Source: CAD feature listing. Evaluate the final solid. Frame: model axes, mm. Face numbers are marked on the shaded views. A direction names the side the tool comes from. Coordinates: 2 decimals unless noted, no trailing zeros. Loops run counter-clockwise (first coordinate to the right, second up) from the corner with the lowest first, then second, coordinate; pieces in that order, holes last.
```python
from build123d import *

# Parameters (mm, degrees)
SM_BASE_FLANGE_1_DEPTH            = 5
SM_EDGE_FLANGE_1_STRIP_W          = 26
SM_EDGE_FLANGE_1_STRIP_H          = 5
SM_EDGE_FLANGE_1_STRIP_CUT_DEPTH  = 45
SM_EDGE_FLANGE_1_RELIEF_W         = 28.5
SM_EDGE_FLANGE_1_RELIEF_H         = 2.5
SM_EDGE_FLANGE_1_RELIEF_CUT_DEPTH = 5
SM_EDGE_FLANGE_1_DEPTH            = 45
SM_EDGE_FLANGE_2_STRIP_W          = 26
SM_EDGE_FLANGE_2_STRIP_H          = 5
SM_EDGE_FLANGE_2_STRIP_CUT_DEPTH  = 45
SM_EDGE_FLANGE_2_RELIEF_W         = 28.5
SM_EDGE_FLANGE_2_RELIEF_H         = 2.5
SM_EDGE_FLANGE_2_RELIEF_CUT_DEPTH = 5
SM_EDGE_FLANGE_2_DEPTH            = 45
SM_EDGE_FLANGE_14_DEPTH           = 40
SM_EDGE_FLANGE_15_DEPTH           = 40
SM_EDGE_FLANGE_16_DEPTH           = 40
SM_EDGE_FLANGE_17_DEPTH           = 40
SM_EDGE_FLANGE_18_STRIP_W         = 26
SM_EDGE_FLANGE_18_STRIP_H         = 5
SM_EDGE_FLANGE_18_STRIP_CUT_DEPTH = 40
SM_EDGE_FLANGE_18_DEPTH           = 40
SM_EDGE_FLANGE_19_STRIP_W         = 26
SM_EDGE_FLANGE_19_STRIP_H         = 5
SM_EDGE_FLANGE_19_STRIP_CUT_DEPTH = 40
SM_EDGE_FLANGE_19_DEPTH           = 40
SM_EDGE_FLANGE_20_STRIP_W         = 26
SM_EDGE_FLANGE_20_STRIP_H         = 5
SM_EDGE_FLANGE_20_STRIP_CUT_DEPTH = 40
SM_EDGE_FLANGE_20_DEPTH           = 40
SM_EDGE_FLANGE_21_STRIP_W         = 26
SM_EDGE_FLANGE_21_STRIP_H         = 5
SM_EDGE_FLANGE_21_STRIP_CUT_DEPTH = 40
SM_EDGE_FLANGE_21_DEPTH           = 40
CUT_EXTRUDE_START                 = -35
SKETCH_80_R                       = 3
CUT_EXTRUDE_1_DEPTH               = 5
CUT_EXTRUDE_3_DEPTH               = 124.060960503
CUT_EXTRUDE_3_DEPTH_BACK          = 124.060960503
SKETCH_83_R                       = 3
CUT_EXTRUDE_START_2               = -30
SKETCH_84_R                       = 3
CUT_EXTRUDE_5_DEPTH               = 5


# Sheet-metal steps are written as plain solids
with BuildPart() as part:
    # Sketch 1 → 基体-法兰1 (new body)
    with BuildSketch(Plane(origin=(0, 0, 0), x_dir=(1, 0, 0), z_dir=(0, 1, 0))):
        Polygon((-25, -25), (-25, -50), (-50, -50), (-50, 50), (-25, 50), (-25, 25), (25, 25), (25, 50), (50, 50), (50, -50), (25, -50), (25, -25), align=None)
    extrude(amount=-SM_BASE_FLANGE_1_DEPTH)

    # 边线-法兰1 strip (across the edge) → 边线-法兰1 strip cut (cut)
    with BuildSketch(Plane(origin=(22.5, 0, -25), x_dir=(0, 0, 1), z_dir=(-1, 0, 0))):
        with Locations((-10, -2.5)):
            Rectangle(SM_EDGE_FLANGE_1_STRIP_W, SM_EDGE_FLANGE_1_STRIP_H)
    extrude(amount=SM_EDGE_FLANGE_1_STRIP_CUT_DEPTH, mode=Mode.SUBTRACT)

    # 边线-法兰1 relief (on the sheet) → 边线-法兰1 relief cut (cut)
    with BuildSketch(Plane(origin=(22.5, 0, -22), x_dir=(0, 0, 1), z_dir=(0, 1, 0))):
        with Locations((-11.75, 1.25)):
            Rectangle(SM_EDGE_FLANGE_1_RELIEF_W, SM_EDGE_FLANGE_1_RELIEF_H)
        with Locations((-11.75, -46.25)):
            Rectangle(SM_EDGE_FLANGE_1_RELIEF_W, SM_EDGE_FLANGE_1_RELIEF_H)
    extrude(amount=-SM_EDGE_FLANGE_1_RELIEF_CUT_DEPTH, mode=Mode.SUBTRACT)

    # 边线-法兰1 section (across the edge) → 边线-法兰1 (add)
    with BuildSketch(Plane(origin=(22.5, 0, -25), x_dir=(0, 0, 1), z_dir=(-1, 0, 0))):
        with BuildLine():
            Line((-5, 3), (-5, 70))
            Line((-5, 70), (0, 70))
            Line((0, 70), (0, 3))
            ThreePointArc((0, 3), (0.878679656, 0.878679656), (3, 0))
            Line((3, 0), (3, -5))
            ThreePointArc((3, -5), (-2.656854249, -2.656854249), (-5, 3))
        make_face()
    extrude(amount=SM_EDGE_FLANGE_1_DEPTH)

    # 边线-法兰2 strip (across the edge) → 边线-法兰2 strip cut (cut)
    with BuildSketch(Plane(origin=(-22.5, 0, 25), x_dir=(0, 0, -1), z_dir=(1, 0, 0))):
        with Locations((-10, -2.5)):
            Rectangle(SM_EDGE_FLANGE_2_STRIP_W, SM_EDGE_FLANGE_2_STRIP_H)
    extrude(amount=SM_EDGE_FLANGE_2_STRIP_CUT_DEPTH, mode=Mode.SUBTRACT)

    # 边线-法兰2 relief (on the sheet) → 边线-法兰2 relief cut (cut)
    with BuildSketch(Plane(origin=(-22.5, 0, 22), x_dir=(0, 0, -1), z_dir=(0, 1, 0))):
        with Locations((-11.75, 1.25)):
            Rectangle(SM_EDGE_FLANGE_2_RELIEF_W, SM_EDGE_FLANGE_2_RELIEF_H)
        with Locations((-11.75, -46.25)):
            Rectangle(SM_EDGE_FLANGE_2_RELIEF_W, SM_EDGE_FLANGE_2_RELIEF_H)
    extrude(amount=-SM_EDGE_FLANGE_2_RELIEF_CUT_DEPTH, mode=Mode.SUBTRACT)

    # 边线-法兰2 section (across the edge) → 边线-法兰2 (add)
    with BuildSketch(Plane(origin=(-22.5, 0, 25), x_dir=(0, 0, -1), z_dir=(1, 0, 0))):
        with BuildLine():
            Line((-5, 3), (-5, 70))
            Line((-5, 70), (0, 70))
            Line((0, 70), (0, 3))
            ThreePointArc((0, 3), (0.878679656, 0.878679656), (3, 0))
            Line((3, 0), (3, -5))
            ThreePointArc((3, -5), (-2.656854249, -2.656854249), (-5, 3))
        make_face()
    extrude(amount=SM_EDGE_FLANGE_2_DEPTH)

    # 边线-法兰14 section (across the edge) → 边线-法兰14 (add)
    with BuildSketch(Plane(origin=(53, -5, 10), x_dir=(-1, 0, 0), z_dir=(0, 0, 1))):
        with BuildLine():
            Line((-5, 3), (-5, 30))
            Line((-5, 30), (0, 30))
            Line((0, 30), (0, 3))
            ThreePointArc((0, 3), (0.878679656, 0.878679656), (3, 0))
            Line((3, 0), (3, -5))
            ThreePointArc((3, -5), (-2.656854249, -2.656854249), (-5, 3))
        make_face()
    extrude(amount=SM_EDGE_FLANGE_14_DEPTH)

    # 边线-法兰15 section (across the edge) → 边线-法兰15 (add)
    with BuildSketch(Plane(origin=(53, -5, -50), x_dir=(-1, 0, 0), z_dir=(0, 0, 1))):
        with BuildLine():
            Line((-5, 3), (-5, 30))
            Line((-5, 30), (0, 30))
            Line((0, 30), (0, 3))
            ThreePointArc((0, 3), (0.878679656, 0.878679656), (3, 0))
            Line((3, 0), (3, -5))
            ThreePointArc((3, -5), (-2.656854249, -2.656854249), (-5, 3))
        make_face()
    extrude(amount=SM_EDGE_FLANGE_15_DEPTH)

    # 边线-法兰16 section (across the edge) → 边线-法兰16 (add)
    with BuildSketch(Plane(origin=(-53, -5, -10), x_dir=(1, 0, 0), z_dir=(0, 0, -1))):
        with BuildLine():
            Line((-5, 3), (-5, 30))
            Line((-5, 30), (0, 30))
            Line((0, 30), (0, 3))
            ThreePointArc((0, 3), (0.878679656, 0.878679656), (3, 0))
            Line((3, 0), (3, -5))
            ThreePointArc((3, -5), (-2.656854249, -2.656854249), (-5, 3))
        make_face()
    extrude(amount=SM_EDGE_FLANGE_16_DEPTH)

    # 边线-法兰17 section (across the edge) → 边线-法兰17 (add)
    with BuildSketch(Plane(origin=(-53, -5, 50), x_dir=(1, 0, 0), z_dir=(0, 0, -1))):
        with BuildLine():
            Line((-5, 3), (-5, 30))
            Line((-5, 30), (0, 30))
            Line((0, 30), (0, 3))
            ThreePointArc((0, 3), (0.878679656, 0.878679656), (3, 0))
            Line((3, 0), (3, -5))
            ThreePointArc((3, -5), (-2.656854249, -2.656854249), (-5, 3))
        make_face()
    extrude(amount=SM_EDGE_FLANGE_17_DEPTH)

    # 边线-法兰18 strip (across the edge) → 边线-法兰18 strip cut (cut)
    with BuildSketch(Plane(origin=(-58, -35, -50), x_dir=(0, 1, 0), z_dir=(0, 0, 1))):
        with Locations((-5, -2.5)):
            Rectangle(SM_EDGE_FLANGE_18_STRIP_W, SM_EDGE_FLANGE_18_STRIP_H)
    extrude(amount=SM_EDGE_FLANGE_18_STRIP_CUT_DEPTH, mode=Mode.SUBTRACT)

    # 边线-法兰18 section (across the edge) → 边线-法兰18 (add)
    with BuildSketch(Plane(origin=(-58, -35, -50), x_dir=(0, 1, 0), z_dir=(0, 0, 1))):
        with BuildLine():
            Line((0, 3), (0, 30))
            Line((0, 30), (5, 30))
            Line((5, 30), (5, 3))
            ThreePointArc((5, 3), (5.878679656, 0.878679656), (8, 0))
            Line((8, 0), (8, -5))
            ThreePointArc((8, -5), (2.343145751, -2.656854249), (0, 3))
        make_face()
    extrude(amount=SM_EDGE_FLANGE_18_DEPTH)

    # 边线-法兰19 strip (across the edge) → 边线-法兰19 strip cut (cut)
    with BuildSketch(Plane(origin=(-58, -35, 10), x_dir=(0, 1, 0), z_dir=(0, 0, 1))):
        with Locations((-5, -2.5)):
            Rectangle(SM_EDGE_FLANGE_19_STRIP_W, SM_EDGE_FLANGE_19_STRIP_H)
    extrude(amount=SM_EDGE_FLANGE_19_STRIP_CUT_DEPTH, mode=Mode.SUBTRACT)

    # 边线-法兰19 section (across the edge) → 边线-法兰19 (add)
    with BuildSketch(Plane(origin=(-58, -35, 10), x_dir=(0, 1, 0), z_dir=(0, 0, 1))):
        with BuildLine():
            Line((0, 3), (0, 30))
            Line((0, 30), (5, 30))
            Line((5, 30), (5, 3))
            ThreePointArc((5, 3), (5.878679656, 0.878679656), (8, 0))
            Line((8, 0), (8, -5))
            ThreePointArc((8, -5), (2.343145751, -2.656854249), (0, 3))
        make_face()
    extrude(amount=SM_EDGE_FLANGE_19_DEPTH)

    # 边线-法兰20 strip (across the edge) → 边线-法兰20 strip cut (cut)
    with BuildSketch(Plane(origin=(58, -35, 50), x_dir=(0, 1, 0), z_dir=(0, 0, -1))):
        with Locations((-5, -2.5)):
            Rectangle(SM_EDGE_FLANGE_20_STRIP_W, SM_EDGE_FLANGE_20_STRIP_H)
    extrude(amount=SM_EDGE_FLANGE_20_STRIP_CUT_DEPTH, mode=Mode.SUBTRACT)

    # 边线-法兰20 section (across the edge) → 边线-法兰20 (add)
    with BuildSketch(Plane(origin=(58, -35, 50), x_dir=(0, 1, 0), z_dir=(0, 0, -1))):
        with BuildLine():
            Line((0, 3), (0, 30))
            Line((0, 30), (5, 30))
            Line((5, 30), (5, 3))
            ThreePointArc((5, 3), (5.878679656, 0.878679656), (8, 0))
            Line((8, 0), (8, -5))
            ThreePointArc((8, -5), (2.343145751, -2.656854249), (0, 3))
        make_face()
    extrude(amount=SM_EDGE_FLANGE_20_DEPTH)

    # 边线-法兰21 strip (across the edge) → 边线-法兰21 strip cut (cut)
    with BuildSketch(Plane(origin=(58, -35, -10), x_dir=(0, 1, 0), z_dir=(0, 0, -1))):
        with Locations((-5, -2.5)):
            Rectangle(SM_EDGE_FLANGE_21_STRIP_W, SM_EDGE_FLANGE_21_STRIP_H)
    extrude(amount=SM_EDGE_FLANGE_21_STRIP_CUT_DEPTH, mode=Mode.SUBTRACT)

    # 边线-法兰21 section (across the edge) → 边线-法兰21 (add)
    with BuildSketch(Plane(origin=(58, -35, -10), x_dir=(0, 1, 0), z_dir=(0, 0, -1))):
        with BuildLine():
            Line((0, 3), (0, 30))
            Line((0, 30), (5, 30))
            Line((5, 30), (5, 3))
            ThreePointArc((5, 3), (5.878679656, 0.878679656), (8, 0))
            Line((8, 0), (8, -5))
            ThreePointArc((8, -5), (2.343145751, -2.656854249), (0, 3))
        make_face()
    extrude(amount=SM_EDGE_FLANGE_21_DEPTH)

    # 草图80 → 切除-拉伸1 (cut)
    with BuildSketch(Plane(origin=(0, 0, 0), x_dir=(1, 0, 0), z_dir=(0, 1, 0)).offset(CUT_EXTRUDE_START)):
        with Locations(Location((-75, 40, 0), (0, 0, 270))):
            Circle(SKETCH_80_R)
        with Locations(Location((75, 40, 0), (0, 0, 270))):
            Circle(SKETCH_80_R)
        with Locations(Location((-75, -40, 0), (0, 0, 270))):
            Circle(SKETCH_80_R)
        with Locations(Location((75, -40, 0), (0, 0, 270))):
            Circle(SKETCH_80_R)
    extrude(amount=CUT_EXTRUDE_1_DEPTH, mode=Mode.SUBTRACT)

    # 草图83 → 切除-拉伸3 (cut, two sides: drawn at the far end of the back side and taken through both)
    with BuildSketch(Plane.XY.offset(-CUT_EXTRUDE_3_DEPTH_BACK)):
        with Locations((0, 50)):
            Circle(SKETCH_83_R)
        with Locations((0, 30)):
            Circle(SKETCH_83_R)
    extrude(amount=CUT_EXTRUDE_3_DEPTH + CUT_EXTRUDE_3_DEPTH_BACK, mode=Mode.SUBTRACT)

    # 草图84 → 切除-拉伸5 (cut)
    with BuildSketch(Plane(origin=(0, 0, 0), x_dir=(1, 0, 0), z_dir=(0, 1, 0)).offset(CUT_EXTRUDE_START_2)):
        with Locations(Location((75, 22.5, 0), (0, 0, 270))):
            Circle(SKETCH_84_R)
        with Locations(Location((75, -22.5, 0), (0, 0, 270))):
            Circle(SKETCH_84_R)
        with Locations(Location((-75, -22.5, 0), (0, 0, 270))):
            Circle(SKETCH_84_R)
        with Locations(Location((-75, 22.5, 0), (0, 0, 270))):
            Circle(SKETCH_84_R)
    extrude(amount=-CUT_EXTRUDE_5_DEPTH, mode=Mode.SUBTRACT)


solid = part.part
```
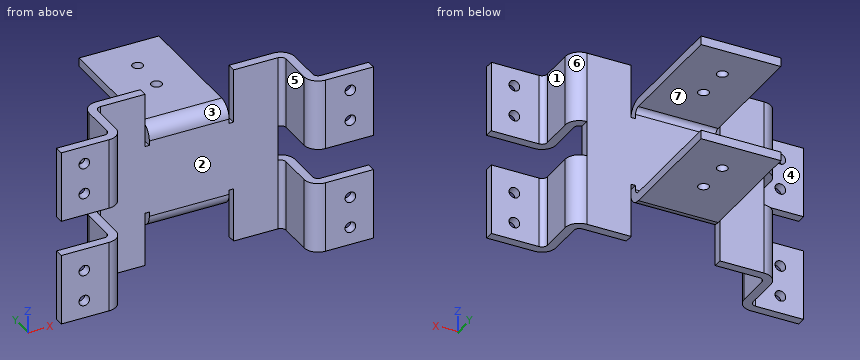
Q1. Section query C-C on z = 40. Count the separate pieces of the cut face and the enclosed holes in it, then the cut area to 3 significant figures.
Q2. Section query B-B on y = 30. Return the cut outline in (x, z), then the cut area to 3 significant figures.
Q3. Material intervals for line 1 along Z through (x, y) = (4.5, 28.5); line 2 along Y through (x, z) = (0, -28.55); line 3 along Y through (x, z) = (0, -28.5), sorted ascending.
Q4. Section query A-A on x = -75. Return the cut outline in (y, z), then the cut area to 3 significant figures.
Q5. Draft query along X for the marked faces 5, 6 and 7. Return one class per face: released by +X, released by -X, zero draft, split by the parting line, or undercut.
Q6. First-contact query: pin 1 Ø6 at (x, z) = (13.5, 2.5) entering from +Y; pin 2 Ø5.5 at (y, z) = (-14, 31.5) entering from -X; pin 3 Ø1 at (y, z) = (-5.5, -19.5) entering from +X. Flat tips, straight axial feed; report the tip coordinate or a pass-through.
Q7. Section query D-D on x = 0. Return the cut outline in (y, z).
Q8. Reachability of the marked faces 1, 2, 3 and 4 from +Z, -Z, +X, -X, +Y, -Y: full face, straight path, thin tool, end or side. Return the list, or none.
Resolved:
1. separate pieces: 4
1. enclosed holes: 0
1. area: 823 mm2
2. outline: (-22.5, -30) - (-3, -30) - (-3, -25) - (-22.5, -25) - close; (-22.5, 25) - (-3, 25) - (-3, 30) - (-22.5, 30) - close; (3, -30) - (22.5, -30) - (22.5, -25) - (3, -25) - close; (3, 25) - (22.5, 25) - (22.5, 30) - (3, 30) - close
2. area: 390 mm2
3. line 1: z = -30 to -25, 25 to 30
3. line 2: y = -1.59 to 27, 33 to 47, 53 to 70
3. line 3: y = -1.66 to 27, 33 to 47, 53 to 70
4. outline: (-35, -50) - (-30, -50) - (-30, -43) - (-35, -43) - close; (-35, -37) - (-30, -37) - (-30, -25.5) - (-35, -25.5) - close; (-35, -19.5) - (-30, -19.5) - (-30, -10) - (-35, -10) - close; (-35, 10) - (-30, 10) - (-30, 19.5) - (-35, 19.5) - close; (-35, 25.5) - (-30, 25.5) - (-30, 37) - (-35, 37) - close; (-35, 43) - (-30, 43) - (-30, 50) - (-35, 50) - close
4. area: 280 mm2
5. face 5: undercut
5. face 6: released by +X
5. face 7: zero draft
6. pin 1: stops at y = 0
6. pin 2: stops at x = -58
6. pin 3: stops at x = 57.75
7. outline: (-5, -22) arc R8 ccw to (3, -30) - (27, -30) - (27, -25) - (3, -25) arc R3 cw to (0, -22) - (0, 22) arc R3 cw to (3, 25) - (27, 25) - (27, 30) - (3, 30) arc R8 ccw to (-5, 22) - close; (33, -30) - (47, -30) - (47, -25) - (33, -25) - close; (33, 25) - (47, 25) - (47, 30) - (33, 30) - close; (53, -30) - (70, -30) - (70, -25) - (53, -25) - close; (53, 25) - (70, 25) - (70, 30) - (53, 30) - close
8. face 1: +Z, -Z, +X, +Y
8. face 2: +Z, -Z, -Y
8. face 3: +Z, -Y
8. face 4: +Z, -Z, -X, +Y
